For this review, take the finished solid that the model builds, in its own axes (mm). Round coordinates to 2 decimals unless told otherwise and drop trailing zeros. Loops run counter-clockwise (first coordinate to the right, second up) from the corner with the lowest first, then second, coordinate; pieces in that order, holes last. Notation, with made-up numbers: (66, -33) -> (87, -33) arc R29 cw to (87, 0) -> close; hole circle Ø6 at (75.25, 61). An arc over 180 degrees is marked (long way). Use one line per item in the form item = value. Start each with the question number.
from build123d import *

# Parameters (mm, degrees)
SKETCH_1_R          = 16.85
SKETCH_1_R_2        = 1.6
SKETCH_1_R_3        = 4.6
EXTRUDE_1_DEPTH     = 2
SKETCH_2_R          = 1.6
CUT_EXTRUDE_1_DEPTH = 3


with BuildPart() as part:
    # 草图1 → 凸台-拉伸1 (new body)
    with BuildSketch(Plane.XY):
        Circle(SKETCH_1_R)
        with Locations((-4.949747468, 4.949747468)):
            Circle(SKETCH_1_R_2, mode=Mode.SUBTRACT)
        with Locations((-4.949747468, -4.949747468)):
            Circle(SKETCH_1_R_2, mode=Mode.SUBTRACT)
        with Locations((4.949747468, -4.949747468)):
            Circle(SKETCH_1_R_2, mode=Mode.SUBTRACT)
        with Locations((4.949747468, 4.949747468)):
            Circle(SKETCH_1_R_2, mode=Mode.SUBTRACT)
        Circle(SKETCH_1_R_3, mode=Mode.SUBTRACT)
    extrude(amount=EXTRUDE_1_DEPTH)

    # 草图2 → 切除-拉伸1 (cut, through all)
    with BuildSketch(Plane(origin=(0, 0, 0), x_dir=(-1, 0, 0), z_dir=(0, 0, -1))):
        with BuildLine():
            ThreePointArc((0, 14.6), (-1.6, 13), (0, 11.4))
            Line((0, 11.4), (0, 14.6))
        make_face()
        with BuildLine():
            Line((0, 14.6), (0, 11.4))
            ThreePointArc((0, 11.4), (1.13137085, 11.86862915), (1.6, 13))
            ThreePointArc((1.6, 13), (1.13137085, 14.13137085), (0, 14.6))
        make_face()
        with Locations((-11.258330249, -6.5)):
            Circle(SKETCH_2_R)
        with Locations((11.258330249, -6.5)):
            Circle(SKETCH_2_R)
    extrude(amount=-CUT_EXTRUDE_1_DEPTH, mode=Mode.SUBTRACT)


solid = part.part
Item 1: Take a section at B-B on x = 11. Give the boundary of the cut face in (y, z), plus the area to 3 significant figures.
Item 2: For P1, Ø12, axis at x = -11, y = -6, coming from the -Z side; P2, Ø1, axis at y = 11.5, z = 0.5, coming from the -X side; P3, Ø1, axis at y = 6, z = 0.5, coming from the +X side, all flat-tipped, find the tip position at first contact; note any pin that passes through.
Item 3: Take a section at C-C on z = 0.95. Give the number of separate pieces and of enclosed holes in the cut face, plus the area to 3 significant figures.
Item 4: Wall thickness on line 1 (Y direction, x = 5, z = 1.7); line 2 (Y direction, x = 6, z = 0.85); line 3 (X direction, y = -7, z = 1.3): over which ranges is each line inside the solid? List them lowest first.
Item 5: Take a section at D-D on y = 10.5. Give the boundary of the cut face in (x, z).
Item 6: Take a section at A-A on y = 0. Give the boundary of the cut face in (x, z).
Item 7: Draft analysis for pull direction X (two halves, no side actions). For faces 1 (the cylindrical face through (12.53, -7.47, 0.99)), 2 (the flat face through (3.5, -3.5, 0)), 3 (the cylindrical face through (-2.194, 16.707, 0.986)), state which applies: +X half, -X half, draft (parallel to the pull), parting line (faces both ways), or undercut.
Results:
q1.outline = (-12.76, 0) -> (-8.08, 0) -> (-8.08, 2) -> (-12.76, 2) -> close; (-4.92, 0) -> (12.76, 0) -> (12.76, 2) -> (-4.92, 2) -> close
q1.area = 44.7 mm2
q2.P1 = 0
q2.P2 = -12.76
q2.P3 = 15.93
q3.separate_pieces = 1
q3.enclosed_holes = 8
q3.area = 769 mm2
q4.line_1 = -16.09 to -6.55, -3.35 to 3.35, 6.55 to 16.09
q4.line_2 = -15.75 to -6.16, -3.74 to 3.74, 6.16 to 15.75
q4.line_3 = -15.33 to -12.78, -9.74 to 9.74, 12.78 to 15.33
q5.outline = (-13.18, 0) -> (13.18, 0) -> (13.18, 2) -> (-13.18, 2) -> close
q6.outline = (-16.85, 0) -> (-4.6, 0) -> (-4.6, 2) -> (-16.85, 2) -> close; (4.6, 0) -> (16.85, 0) -> (16.85, 2) -> (4.6, 2) -> close
q7.face_1 = undercut
q7.face_2 = draft
q7.face_3 = parting line
